The figure shows three views and two pictorial views of one solid part (mm, origin at its lowest corner). Answer the questions. Coordinates: 2 decimals unless noted, no trailing zeros. Loops run counter-clockwise (first coordinate to the right, second up) from the corner with the lowest first, then second, coordinate; pieces in that order, holes last.
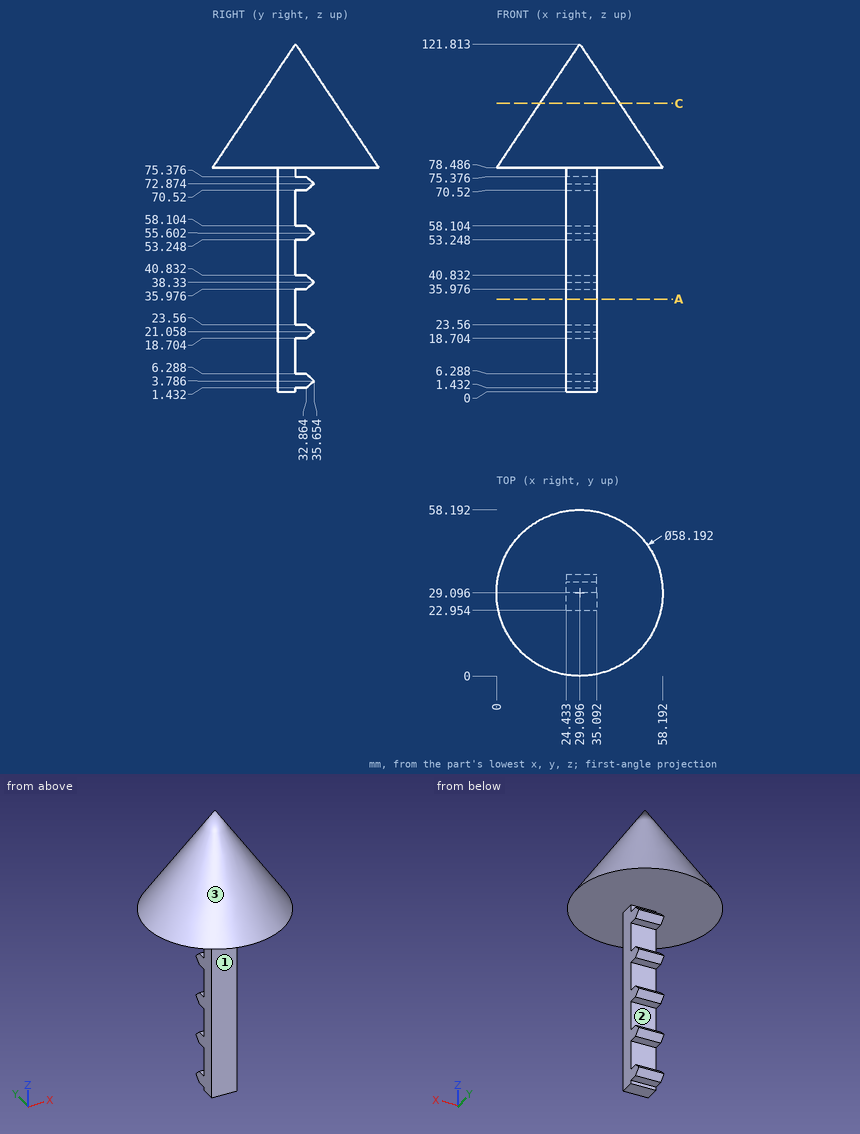
1. A cutting plane is placed at A-A, the plane z = 32.5. Give the vertices of the cut face in (x, y) (1 decimal).
2. Determine the mould class of the marked faces 1, 2 and 3 for opening direction Z: released by +Z, released by -Z, zero draft, split by the parting line, or undercut.
3. A cutting plane is placed at C-C, the plane z = 101. Give the vertices of the cut face in (x, y) (1 decimal), then the cut area to 3 significant figures.
4. Each of these flat-tipped pins is pushed along its axis until it touches: P1, Ø4, axis at x = 11, y = 11, coming from the -Z side; P2, Ø3, axis at x = 29.5, z = 27.5, coming from the +Y side; P3, Ø5.5, axis at x = 27.5, z = 53, coming from the -Y side. Where does it stop, or does it pass through?
5. Straight lines are drawn through the part: probe 1 along X at (y, z) = (24, 14); probe 2 along Z at (x, y) = (40, 10.5) (1 decimal); probe 3 along Z at (x, y) = (23, 21) (1 decimal). For each, find the intervals that lie inside material, in ascending order.
Answers below:
1. outline: (24.4, 23) - (35.1, 23) - (35.1, 29.1) - (24.4, 29.1) - close
2. face 1: zero draft
2. face 2: undercut
2. face 3: released by +Z
3. outline: circle Ø28 at (29.1, 29.1)
3. area: 614 mm2
4. P1: stops at z = 78.49
4. P2: stops at y = 29.1
4. P3: stops at y = 22.95
5. probe 1: x = 24.43 to 35.09
5. probe 2: z = 78.5 to 89.7
5. probe 3: z = 78.5 to 106.7
